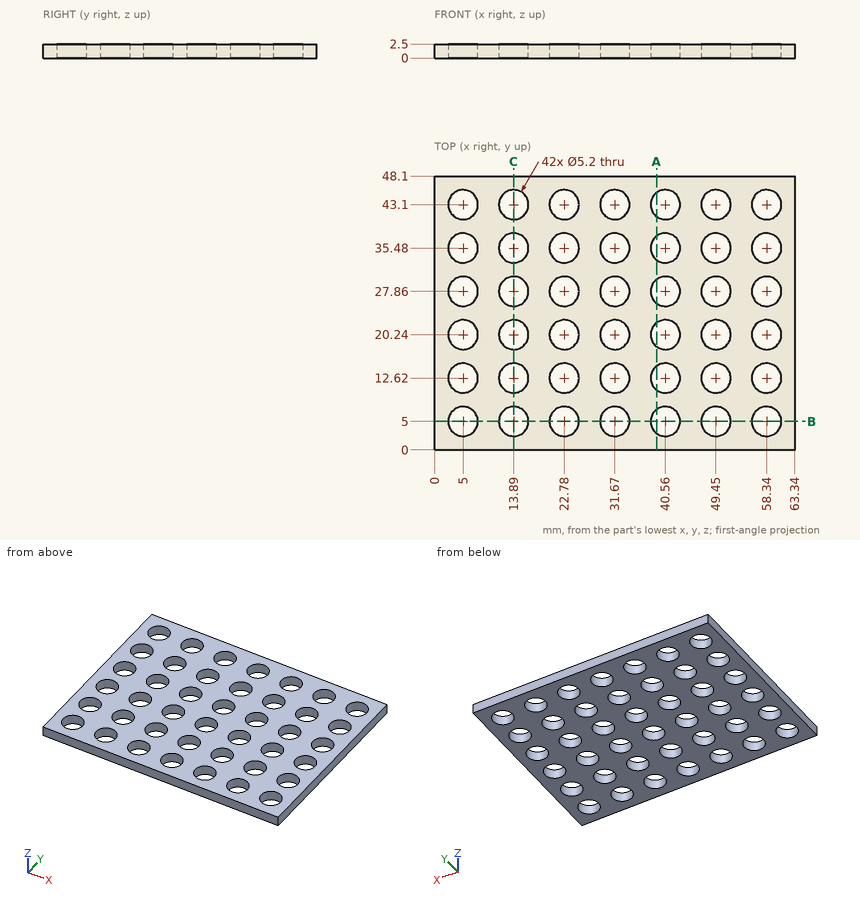
Design review of the part shown in the three views and the two pictorial views. Dimensions are in mm from the part's minimum x, y and z. Round coordinates to 2 decimals unless told otherwise and drop trailing zeros. Write each loop counter-clockwise with the first axis right and the second up, starting at its lowest first coordinate (ties: lowest second). Pieces come first, ordered by that corner, then holes. Notation, with made-up numbers: (85.5, -38) - (111.5, -38) arc R29 ccw to (111.5, -11) - close; hole circle Ø5 at (-38.5, 20). An arc over 180 degrees is marked (long way). Answer as CSV lines item,"result". Start each with the question number.
(1) Add section C-C, the plane x = 13.89. State the section outline as (y, z) points.
(2) Add section A-A, the plane x = 39. State the section outline as (y, z) points, plus the area to 4 significant figures.
(3) Add section B-B, the plane y = 5. State how many separate pieces and enclosed holes the cut face has, plus the area to 4 significant figures.
(4) For pin 1 (4 mm diameter, centred on x = 49.45, y = 5, fed in from -Z), flat-tipped, find the tip position at first contact; note if it passes through.
From the geometry:
1,outline,"(0, 0) - (2.4, 0) - (2.4, 2.5) - (0, 2.5) - close; (7.6, 0) - (10.02, 0) - (10.02, 2.5) - (7.6, 2.5) - close; (15.22, 0) - (17.64, 0) - (17.64, 2.5) - (15.22, 2.5) - close; (22.84, 0) - (25.26, 0) - (25.26, 2.5) - (22.84, 2.5) - close; (30.46, 0) - (32.88, 0) - (32.88, 2.5) - (30.46, 2.5) - close; (38.08, 0) - (40.5, 0) - (40.5, 2.5) - (38.08, 2.5) - close; (45.7, 0) - (48.1, 0) - (48.1, 2.5) - (45.7, 2.5) - close"
2,outline,"(0, 0) - (2.92, 0) - (2.92, 2.5) - (0, 2.5) - close; (7.08, 0) - (10.54, 0) - (10.54, 2.5) - (7.08, 2.5) - close; (14.7, 0) - (18.16, 0) - (18.16, 2.5) - (14.7, 2.5) - close; (22.32, 0) - (25.78, 0) - (25.78, 2.5) - (22.32, 2.5) - close; (29.94, 0) - (33.4, 0) - (33.4, 2.5) - (29.94, 2.5) - close; (37.56, 0) - (41.02, 0) - (41.02, 2.5) - (37.56, 2.5) - close; (45.18, 0) - (48.1, 0) - (48.1, 2.5) - (45.18, 2.5) - close"
2,area,"57.85 mm²"
3,separate pieces,"8"
3,enclosed holes,"0"
3,area,"67.35 mm²"
4,pin 1,"passes through"
